from build123d import *

# Parameters (mm, degrees)
CUT_EXTRUDE_1_DEPTH         = 20
SKETCH_4_R                  = 2
SKETCH_4_R_2                = 30
CUT_EXTRUDE_2_DEPTH         = 47.647615159
FILLET_1_R                  = 3
SKETCH_5_R                  = 2
SKETCH_5_R_2                = 1.5
CUT_EXTRUDE_3_DEPTH         = 20
CUT_EXTRUDE_5_DEPTH         = 8.5
SKETCH_9_R                  = 1.5
CUT_EXTRUDE_6_DEPTH         = 51.644290358
SKETCH_11_R                 = 8
CUT_EXTRUDE_8_DEPTH         = 5
HOLE_WIZARD_12_0_12_1_D     = 12
HOLE_WIZARD_12_0_12_1_DEPTH = 10
HOLE_WIZARD_12_0_12_1_TIP   = 3.605163714
FILLET_2_R                  = 0.6
CHAMFER_2_SIZE              = 0.5
CHAMFER_2_SIZE2             = 0.288675135
CHAMFER_3_SIZE              = 0.5
CHAMFER_3_SIZE2             = 0.288675135


with BuildPart() as part:
    # 草图2 → 旋转1 (revolve)
    with BuildSketch(Plane.XY, mode=Mode.PRIVATE) as revolve_1_sk:
        Polygon((-7.5, 0), (-7.5, 15), (-8.5, 15), (-8.5, 22), (-9.3, 22), (-9.3, 32), (-24, 32), (-24, 35), (-8, 35), (-8, 40), (-5, 40), (0, 40), (0, 0), (-5, 0), align=None)
    revolve(revolve_1_sk.sketch.rotate(Axis((0, 41.059829881, 0), (0, -1, 0)), 270), axis=Axis((0, 41.059829881, 0), (0, -1, 0)))

    # 草图3 → 切除-拉伸1 (cut)
    with BuildSketch(Plane.XZ):
        with BuildLine():
            Line((-3, 4), (3, 4))
            ThreePointArc((3, 4), (0, -5), (-3, 4))
        make_face()
    extrude(amount=-CUT_EXTRUDE_1_DEPTH, mode=Mode.SUBTRACT)

    # 草图4 → 切除-拉伸2 (cut, through all)
    with BuildSketch(Plane.XZ.offset(-32)):
        with Locations(Location((0, 20, 0), (0, 0, 270))):
            Circle(SKETCH_4_R)
        with Locations(Location((17.320508076, -10, 0), (0, 0, 270))):
            Circle(SKETCH_4_R)
        with Locations(Location((-17.320508076, -10, 0), (0, 0, 270))):
            Circle(SKETCH_4_R)
        with Locations((0, -40)):
            Circle(SKETCH_4_R_2)
        with Locations((-34.641016151, 20)):
            Circle(SKETCH_4_R_2)
        with Locations((34.641016151, 20)):
            Circle(SKETCH_4_R_2)
    extrude(amount=-CUT_EXTRUDE_2_DEPTH, mode=Mode.SUBTRACT)

    # 圆角1
    fillet_1_edges = [part.edges().sort_by_distance(p)[0] for p in [
        (-4.846535333, 33.5, 23.505554562),
        (-22.779675047, 33.5, -7.555554562),
        (-17.933139714, 33.5, -15.95),
        (17.933139714, 33.5, -15.95),
        (22.779675047, 33.5, -7.555554562),
        (4.846535333, 33.5, 23.505554562),
    ]]
    fillet(fillet_1_edges, radius=FILLET_1_R)

    # 草图5 → 切除-拉伸3 (cut)
    with BuildSketch(Plane.XY):
        with Locations(Location((0, 4, 0), (0, 0, 90))):
            Circle(SKETCH_5_R)
        with Locations(Location((0, 10, 0), (0, 0, 90))):
            Circle(SKETCH_5_R_2)
    extrude(amount=CUT_EXTRUDE_3_DEPTH, mode=Mode.SUBTRACT)

    # 草图8 → 切除-拉伸5 (cut)
    with BuildSketch(Plane.XZ.offset(-15)):
        with BuildLine():
            Line((-2.5, 7.071067812), (2.5, 7.071067812))
            ThreePointArc((2.5, 7.071067812), (0, 7.5), (-2.5, 7.071067812))
        make_face()
        with BuildLine():
            Line((-2.5, -7.071067812), (2.5, -7.071067812))
            ThreePointArc((2.5, -7.071067812), (0, -7.5), (-2.5, -7.071067812))
        make_face()
    extrude(amount=CUT_EXTRUDE_5_DEPTH, mode=Mode.SUBTRACT)

    # 草图9 → 切除-拉伸6 (cut, through all)
    with BuildSketch(Plane.XY.offset(7.071067812)):
        with Locations((0, 10)):
            Circle(SKETCH_9_R)
    extrude(amount=-CUT_EXTRUDE_6_DEPTH, mode=Mode.SUBTRACT)

    # 草图11 → 切除-拉伸8 (cut)
    with BuildSketch(Plane(origin=(0, 40, 0), x_dir=(1, 0, 0), z_dir=(0, 1, 0))):
        Circle(SKETCH_11_R)
    extrude(amount=-CUT_EXTRUDE_8_DEPTH, mode=Mode.SUBTRACT)

    # Ø12.0 (12) 直径孔1
    with Locations(Plane.ZX.offset(35)):
        with Locations((0, 0)):
            Hole(HOLE_WIZARD_12_0_12_1_D / 2, depth=HOLE_WIZARD_12_0_12_1_DEPTH)
            with Locations((0, 0, -(HOLE_WIZARD_12_0_12_1_DEPTH + HOLE_WIZARD_12_0_12_1_TIP / 2))):  # 118° drill point
                Cone(0, HOLE_WIZARD_12_0_12_1_D / 2, HOLE_WIZARD_12_0_12_1_TIP, mode=Mode.SUBTRACT)

    # 圆角2
    fillet_2_edges = [part.edges().sort_by_distance(p)[0] for p in [
        (0, 32, -9.3),
    ]]
    fillet(fillet_2_edges, radius=FILLET_2_R)

    # 倒角2
    chamfer_2_edges = [part.edges().sort_by_distance(p)[0] for p in [
        (0, 15, -8.5),
    ]]
    chamfer_2_side = [part.faces().sort_by_distance(p)[0] for p in [
        (-7.740416306, 15, 0),
    ]]
    chamfer(chamfer_2_edges, length=CHAMFER_2_SIZE, length2=CHAMFER_2_SIZE2, reference=chamfer_2_side[0])

    # 倒角3
    chamfer_3_edges = [part.edges().sort_by_distance(p)[0] for p in [
        (0, 0, -5),
    ]]
    chamfer_3_side = [part.faces().sort_by_distance(p)[0] for p in [
        (0, 0, -7.287867966),
    ]]
    chamfer(chamfer_3_edges, length=CHAMFER_3_SIZE, length2=CHAMFER_3_SIZE2, reference=chamfer_3_side[0])


solid = part.part
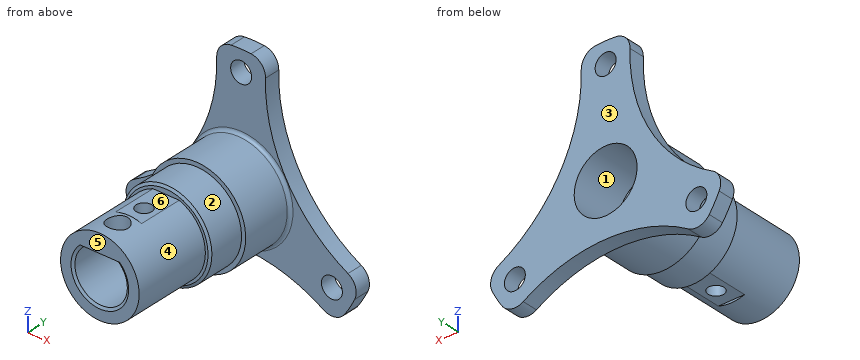
Input: part model. Units: mm. Frame: model coordinates. Face numbers are marked on the shaded views. A direction names the side the tool comes from. Give positions to 0.01 mm unless a question says otherwise; leave off trailing zeros. Loops run counter-clockwise (first coordinate to the right, second up) from the corner with the lowest first, then second, coordinate; pieces in that order, holes last. Notation, with made-up numbers: M -11,-21.5 L 9,-21.5 A12 ccw 9,-10.5 Z; hole C 46.25,3 d10. An arc over 180 degrees is marked long. Use one line per item in the form item = value.
1. Section query B-B, the plane y = 10. Return the cut outline in (x, z), and give its area (3 significant figures).
Numbers:
outline = M -3,4 L -1.5,4 L -1.5,7.07 L -2.5,7.07 A7.5 ccw -2.5,-7.07 L -1.5,-7.07 L -1.5,-4.77 A5 cw Z; M 1.5,-7.07 L 2.5,-7.07 A7.5 ccw 2.5,7.07 L 1.5,7.07 L 1.5,4 L 3,4 A5 cw 1.5,-4.77 Z
area = 83.7 mm²
2. Section query C-C, the plane y = 30. Return the cut outline in (x, z), and give its area (3 significant figures).
Numbers:
outline = C 0,0 d18.6; hole C 0,0 d12
area = 159 mm²
3. Line query: L1, parallel to X at y = 31, z = 0; L2, parallel to Y at x = -16, z = -5; L3, parallel to X at y = 4, z = 6.15. Output: solid intervals per line, ascending.
Numbers:
L1 = -9.3 to -6, 6 to 9.3
L2 = 32 to 35
L3 = -4.29 to -2, 2 to 4.29
4. Section query D-D, the plane x = 14. Return the cut outline in (y, z).
Numbers:
outline = M 32,-13.47 L 35,-13.47 L 35,-1.77 L 32,-1.77 Z
5. First-contact query: pin 1 (1.5 mm diameter, centred on x = 0, y = 9, fed in from -Z); pin 2 (4 mm diameter, centred on y = 28, z = -1.5, fed in from +X); pin 3 (2.5 mm diameter, centred on x = -1, y = 11, fed in from +Z). Flat tips, straight axial feed; report the tip coordinate or a pass-through.
Numbers:
pin_1 = -7.07
pin_2 = 9.3
pin_3 = 7.07
6. Section query A-A, the plane z = 20. Return the cut outline in (x, y).
Numbers:
outline = M -4.64,32 L -2,32 L -2,35 L -4.64,35 Z; M 2,32 L 4.64,32 L 4.64,35 L 2,35 Z
7. Pull-direction query (Z, two-part tool) for the marked faces 1, 2 and 3; classes: released by +Z, released by -Z, zero draft, split by the parting line, or undercut.
Numbers:
face_1 = undercut
face_2 = split by the parting line
face_3 = zero draft
8. Reachability of the marked faces 4, 5 and 6 from +Z, -Z, +X, -X, +Y, -Y: full face, straight path, thin tool, end or side. Return the list, or none.
Numbers:
face_4 = -Y
face_5 = +Z, -Z, +X, -X, -Y
face_6 = +Z, +X, -X
